```python
from build123d import *

# Parameters (mm, degrees)
F0_W     = 63.5
F0_H     = 44.45
F1_DEPTH = 19.05
F3_DEPTH = 19.05
F4_W     = 44.45
F4_H     = 19.05
F5_DEPTH = 19.05


with BuildPart() as f1:
    # F0 (on Top) → F1 (new body)
    with BuildSketch(Plane.XY):
        with Locations((-31.75, 22.225)):
            Rectangle(F0_W, F0_H)
    extrude(amount=F1_DEPTH)

    # F2 (on Right) → F3 (join)
    with BuildSketch(Plane.YZ):
        Polygon((0, 44.45), (0, 0), (63.5, 0), (63.5, 12.7), (19.05, 44.45), align=None)
    extrude(amount=F3_DEPTH)

    # F4 (on face) → F5 (join)
    with BuildSketch(Plane(origin=(-63.5, 0, 0), x_dir=(0, -1, 0), z_dir=(-1, 0, 0))):
        Polygon((-44.45, 19.05), (0, 19.05), (0, 44.45), (-19.05, 44.45), (-63.5, 19.05), (-63.5, 0), (-44.45, 0), align=None)
        with Locations((-22.225, 9.525)):
            Rectangle(F4_W, F4_H)
    extrude(amount=F5_DEPTH)


solid = f1.part
```
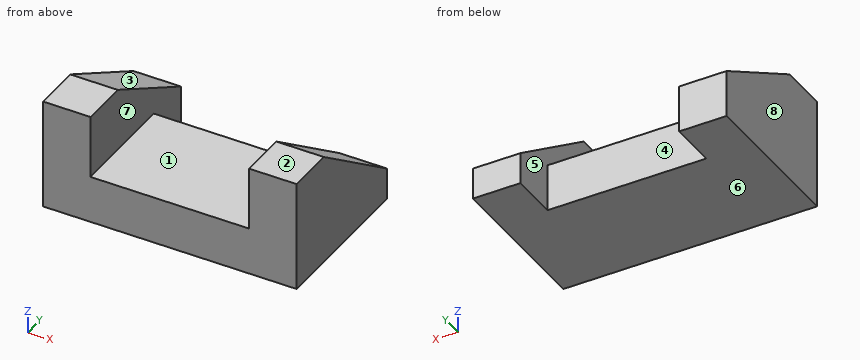
Input: part model. Units: mm. Frame: model coordinates. Face numbers are marked on the shaded views. A direction names the side the tool comes from. Give positions to 0.01 mm unless a question says otherwise; leave off trailing zeros. Loops run counter-clockwise (first coordinate to the right, second up) from the corner with the lowest first, then second, coordinate; pieces in that order, holes last. Notation, with made-up numbers: M 49.5,70.5 L 66.5,70.5 A15 ccw 66.5,75.5 Z; hole C -13,39.25 d3. An arc over 180 degrees is marked long. Answer as CSV lines item,"result". Start each with the question number.
1. Section D-D on y = 10. Return loops of the section in (x, z), plus the area to 3 significant figures.
2. Section A-A on z = 41. Return loops of the section in (x, y), plus the area to 3 significant figures.
3. Section B-B on y = 53.5. Return loops of the section in (x, z), plus the area to 3 significant figures.
4. Pin query (flat end, axial travel): P1, Ø8, axis at x = -26.5, y = 13, coming from the +Z side; P2, Ø15, axis at x = -24, z = 6, coming from the +Y side. Return the tip coordinate at first contact, or that it passes through.
5. Reachability of the marked faces 1, 2, 3, 4 and 5 from +Z, -Z, +X, -X, +Y, -Y: full face, straight path, thin tool, end or side. Return the list, or none.
6. Pull-direction query (X, two-part tool) for the marked faces 6, 7 and 8; classes: released by +X, released by -X, zero draft, split by the parting line, or undercut.
7. Line query: L1, parallel to X at y = 56, z = 4.5; L2, parallel to Z at x = -36, y = 10; L3, parallel to X at y = 31.5, z = 36.5. Output: solid intervals per line, ascending.
8. Section C-C on z = 6.5. Return loops of the section in (x, y), plus the area to 3 significant figures.
Computed values:
1,outline,"M -82.55,0 L 19.05,0 L 19.05,44.45 L 0,44.45 L 0,19.05 L -63.5,19.05 L -63.5,44.45 L -82.55,44.45 Z"
1,area,"2,900 mm²"
2,outline,"M -82.55,0 L -63.5,0 L -63.5,25.09 L -82.55,25.09 Z; M 0,0 L 19.05,0 L 19.05,23.88 L 0,23.88 Z"
2,area,"933 mm²"
3,outline,"M -82.55,0 L -63.5,0 L -63.5,24.76 L -82.55,24.76 Z; M 0,0 L 19.05,0 L 19.05,19.84 L 0,19.84 Z"
3,area,"850 mm²"
4,P1,"stops at z = 19.05"
4,P2,"stops at y = 44.45"
5,face 1,"+Z, +Y, -Y"
5,face 2,"+Z, +X, -X, +Y, -Y"
5,face 3,"+Z, +X, -X, +Y"
5,face 4,"+Z, -Z, +Y"
5,face 5,"+Z, +Y"
6,face 6,"zero draft"
6,face 7,"undercut"
6,face 8,"released by -X"
7,L1,"x = -82.55 to -63.5, 0 to 19.05"
7,L2,"z = 0 to 19.05"
7,L3,"x = -82.55 to -63.5"
8,outline,"M -82.55,0 L 19.05,0 L 19.05,63.5 L 0,63.5 L 0,44.45 L -63.5,44.45 L -63.5,63.5 L -82.55,63.5 Z"
8,area,"5,240 mm²"
